Here's how the part is built. I have some questions about the finished solid (model axes, mm). A direction names the side the tool comes from. Give positions to 0.01 mm unless a question says otherwise; leave off trailing zeros. Write each loop counter-clockwise with the first axis right and the second up, starting at its lowest first coordinate (ties: lowest second). Pieces come first, ordered by that corner, then holes. Notation, with made-up numbers: (53, -19.5) - (108, -19.5) arc R22 ccw to (108, 5.5) - close; hole circle Ø9 at (68, 55). An arc over 180 degrees is marked (long way). One line per item, written item: value. Start each with the question number.
1) Please list where these lines run through material, in increasing order: L1, parallel to Y at x = 32.25, z = -6; L2, parallel to Z at x = 31, y = 154; L3, parallel to Y at x = -13, z = 0. Write a range as [from, to].
2) On a 3-axis mill with a long thin cutter (end or side, diameter ignored), from which of +Z, -Z, +X, -X, +Y, -Y can I reach the whole of each face in a straight line? I mean faces 1 (the flat face through (17, 94, 0)), 2 (the flat face through (-20, 79, 0)), 3 (the flat face through (33, 202, 0)), 4 (the cylindrical face through (32.563, 152.004, -7.038)), 5 (the flat face through (-18, 20, 0)). Say none if no direction works.
3) I'm going to push flat-ended pins straight in: P1, Ø4.5, axis at x = 28, z = -4.5, coming from the -Y side; P2, Ø10, axis at x = 31, y = 189, coming from the +Z side; P3, Ø24, axis at x = -1, z = 0.5, coming from the +Y side. Where does each tip first touch, or does it pass through?
4) We'd pull the mould along X, two halves only. Please class faces 6 (the flat face through (37, 154, 0)), 7 (the flat face through (-15, 145, 12)), 8 (the flat face through (31, 212, 0)), 9 (the cylindrical face through (16.038, 143.004, 16.056)): +X half, -X half, draft (parallel to the pull), parting line (faces both ways), or undercut.
5) Imagine slicing it at A-A on x = 0. Write out the boundary of the cut face in (y, z).
6) Imagine slicing it at C-C on y = 205. Write out the boundary of the cut face in (x, z), plus the area to 3 significant figures.
7) Imagine slicing it at B-B on y = 107.5. Write out the boundary of the cut face in (x, z).
Autodesk Inventor part; units mm, degrees
ref_plane "XZ Plane" through (0, 0, 0) normal (0, 1, 0) x (-1, 0, 0)
ref_plane "XY Plane" through (0, 0, 0) normal (0, 0, 1) x (1, 0, 0)
sketch "スケッチ1" plane through (0, 0, 0) normal (0, 1, 0) x (-1, 0, 0)
  line L0 (16.5, 16.5) -> (-16.5, 16.5)
  line L1 (-16.5, 16.5) -> (-16.5, -16.5)
  line L2 (-16.5, -16.5) -> (16.5, -16.5)
  line L3 (16.5, -16.5) -> (16.5, 16.5)
  line L4 (-23.1, 0) -> (23.1, 0)
  line L5 (0, -23.1) -> (0, 23.1)
  point P0 (0, 0)
  dimension "d0" = 33
  dimension "d1" = 33
extrude "押し出し1" add sketch "スケッチ1" along normal blind 20
fillet "フィレット1" radius 2 4 edges at (16.5, 10, 16.5) (-16.5, 10, 16.5) (16.5, 10, -16.5) (-16.5, 10, -16.5)
sketch "スケッチ2" plane through (0, 20, 0) normal (0, 1, 0) x (1, 0, 0)
  line L0 (-20, -20) -> (20, -20)
  line L1 (20, -20) -> (20, 20)
  line L2 (20, 20) -> (-20, 20)
  line L3 (-20, 20) -> (-20, -20)
  line L4 (-14.5, -16.5) -> (14.5, -16.5)
  line L5 (-16.5, 14.5) -> (-16.5, -14.5)
  line L6 (16.5, -14.5) -> (16.5, 14.5)
  line L7 (14.5, 16.5) -> (-14.5, 16.5)
  point P0 (0, 0)
  dimension "d5" = 3.5
  dimension "d6" = 3.5
  dimension "d7" = 3.5
  dimension "d8" = 3.5
extrude "押し出し2" add sketch "スケッチ2" along normal blind 30
fillet "フィレット2" radius 2 4 edges at (20, 35, 20) (20, 35, -20) (-20, 35, -20) (-20, 35, 20)
sketch "スケッチ3" plane through (0, 0, 0) normal (0, -1, 0) x (1, 0, 0)
  line L0 (12, 14) -> (-12, 14)
  line L1 (-14, 12) -> (-14, -12)
  line L2 (-12, -14) -> (12, -14)
  line L3 (14, -12) -> (14, 12)
  arc A0 (14, 12) -> (12, 14) centre (12, 12) ccw
  arc A1 (12, -14) -> (14, -12) centre (12, -12) ccw
  arc A2 (-14, -12) -> (-12, -14) centre (-12, -12) ccw
  arc A3 (-12, 14) -> (-14, 12) centre (-12, 12) ccw
  line L4 (16.5, 14.5) -> (16.5, -14.5)
  line L5 (14.5, -16.5) -> (-14.5, -16.5)
  line L6 (-14.5, 16.5) -> (14.5, 16.5)
  line L7 (-16.5, -14.5) -> (-16.5, 14.5)
  point P0 (0, 0)
  dimension "d12" = 2
  dimension "d13" = 2.5
  dimension "d14" = 2.5
  dimension "d15" = 2.5
  dimension "d16" = 2.5
extrude "押し出し3" cut sketch "スケッチ3" against normal up to next
sketch "スケッチ4" plane through (0, 50, 0) normal (0, 1, 0) x (1, 0, 0)
  line L0 (18, 20) -> (-18, 20)
  arc A0 (-18, 20) -> (-20, 18) centre (-18, 18) ccw
  line L1 (-20, 18) -> (-20, -18)
  arc A1 (-20, -18) -> (-18, -20) centre (-18, -18) ccw
  line L2 (-18, -20) -> (18, -20)
  arc A2 (18, -20) -> (20, -18) centre (18, -18) ccw
  line L3 (20, -18) -> (20, 18)
  arc A3 (20, 18) -> (18, 20) centre (18, 18) ccw
  line L4 (-15, 17) -> (15, 17)
  line L5 (17, 15) -> (17, -15)
  line L6 (15, -17) -> (-15, -17)
  line L7 (-17, -15) -> (-17, 15)
  arc A4 (-15, 17) -> (-17, 15) centre (-15, 15) ccw
  arc A5 (-17, -15) -> (-15, -17) centre (-15, -15) ccw
  arc A6 (15, -17) -> (17, -15) centre (15, -15) ccw
  arc A7 (17, 15) -> (15, 17) centre (15, 15) ccw
  point P0 (0, 0)
  dimension "d21" = 2
  dimension "d22" = 3
  dimension "d23" = 3
  dimension "d24" = 3
  dimension "d25" = 3
extrude "押し出し5" add sketch "スケッチ4" along normal blind 90
sketch "スケッチ5" plane through (0, 140, 0) normal (0, 1, 0) x (1, 0, 0)
  line L0 (18, 20) -> (-18, 20)
  arc A0 (-18, 20) -> (-20, 18) centre (-18, 18) ccw
  line L1 (-20, 18) -> (-20, -18)
  arc A1 (-20, -18) -> (-18, -20) centre (-18, -18) ccw
  line L2 (-18, -20) -> (18, -20)
  arc A2 (18, -20) -> (20, -18) centre (18, -18) ccw
  line L3 (20, -18) -> (20, 18)
  arc A3 (20, 18) -> (18, 20) centre (18, 18) ccw
  point P0 (0, 0)
extrude "押し出し6" add sketch "スケッチ5" along normal blind 10
sketch "スケッチ6" plane through (0, 150, 0) normal (0, 1, 0) x (1, 0, 0)
  circle A0 centre (0, 0) radius 15
  dimension "d30" = 30
extrude "押し出し7" add sketch "スケッチ6" along normal blind 15
sketch "スケッチ7" plane through (0, 165, 0) normal (0, 1, 0) x (1, 0, 0)
  circle A0 centre (0, 0) radius 12
  circle A1 centre (0, 0) radius 15
  dimension "d33" = 3
extrude "押し出し8" cut sketch "スケッチ7" against normal up to next contours A0
sketch "スケッチ8" plane through (20, 20, 18) normal (1, 0, 0) x (0, 0, -1)
  line L0 (34, 130) -> (2, 130)
  line L1 (2, 130) -> (2, 110)
  line L2 (2, 110) -> (34, 110)
  line L3 (34, 110) -> (34, 130)
  line L4 (0, 130) -> (36, 130)
  line L5 (38, 0) -> (38, 130)
  line L6 (-2, 130) -> (-2, 0)
  point P0 (18, -20)
  dimension "d36" = 20
  dimension "d37" = 32
  dimension "d38" = 4
  dimension "d39" = 4
extrude "押し出し9" add sketch "スケッチ8" along normal blind 8
sketch "スケッチ9" plane through (28, 20, 18) normal (1, 0, 0) x (0, 0, -1)
  line L0 (34, 130) -> (34, 110)
  line L1 (34, 110) -> (2, 110)
  line L2 (2, 110) -> (2, 192)
  line L3 (2, 192) -> (34, 192)
  line L4 (34, 192) -> (34, 110)
  line L5 (34, 130) -> (2, 130)
  point P0 (18, -20)
  dimension "d42" = 32
  dimension "d43" = 62
extrude "押し出し10" add sketch "スケッチ9" along normal blind 9
sketch "スケッチ10" plane through (37, 20, 18) normal (1, 0, 0) x (0, 0, -1)
  line L0 (28.5, 182) -> (7.5, 182)
  line L1 (6.5, 181) -> (6.5, 138)
  line L2 (7.5, 137) -> (28.5, 137)
  line L3 (29.5, 138) -> (29.5, 181)
  line L4 (34, 192) -> (2, 192)
  line L5 (34, 110) -> (34, 192)
  line L6 (2, 192) -> (2, 110)
  arc A0 (29.5, 181) -> (28.5, 182) centre (28.5, 181) ccw
  arc A1 (28.5, 137) -> (29.5, 138) centre (28.5, 138) ccw
  arc A2 (6.5, 138) -> (7.5, 137) centre (7.5, 138) ccw
  arc A3 (7.5, 182) -> (6.5, 181) centre (7.5, 181) ccw
  point P0 (18, -20)
  point P1 (29.5, 182)
  point P2 (6.5, 182)
  point P3 (29.5, 137)
  dimension "d46" = 45
  dimension "d47" = 23
  dimension "d48" = 10
  dimension "d49" = 4.5
  dimension "d50" = 4.5
  dimension "d51" = 1
extrude "押し出し11" cut sketch "スケッチ10" against normal up to next
fillet "フィレット3" radius 2 8 edges at (32.5, 212, -16) (32.5, 212, 16) (28.5, 130, -16) (28.5, 130, 16) (37, 130, 0) (37, 171, -16) (37, 171, 16) (37, 212, 0)
sketch "スケッチ11" plane through (37, 20, 18) normal (1, 0, 0) x (0, 0, -1)
  circle A0 centre (24, 185) radius 2.25
  circle A1 centre (12, 185) radius 2.25
  circle A2 centre (24, 134) radius 2.25
  circle A3 centre (12, 134) radius 2.25
  line L0 (7.5, 182) -> (28.5, 182)
  line L1 (28.5, 137) -> (7.5, 137)
  line L2 (34, 112) -> (34, 190)
  line L3 (2, 190) -> (2, 112)
  point P0 (18, -20)
  point P1 (34, 150)
  point P2 (2, 150)
  dimension "d55" = 12
  dimension "d56" = 4.5
  dimension "d57" = 4.5
  dimension "d58" = 4.5
  dimension "d59" = 4.5
  dimension "d60" = 12
  dimension "d61" = 51
  dimension "d62" = 51
  dimension "d63" = 3
  dimension "d64" = 3
  dimension "d65" = 10
  dimension "d66" = 10
extrude "押し出し12" cut sketch "スケッチ11" against normal up to next contours A0
extrude "押し出し13" cut sketch "スケッチ11" against normal up to next contours A1
extrude "押し出し14" cut sketch "スケッチ11" against normal up to next contours A2
extrude "押し出し15" cut sketch "スケッチ11" against normal up to next contours A3
sketch "スケッチ21" plane through (-18, 20, 20) normal (0, 0, 1) x (1, 0, 0)
  circle A0 centre (3, 125) radius 2.25
  circle A1 centre (33, 125) radius 2.25
  line L0 (0, 0) -> (0, 130)
  line L1 (36, 130) -> (36, 0)
  line L2 (0, 130) -> (36, 130)
  point P0 (18, -20)
  dimension "d122" = 4.5
  dimension "d123" = 4.5
  dimension "d124" = 3
  dimension "d125" = 30
  dimension "d127" = 5
  dimension "d128" = 5
  dimension "d129" = 3
extrude "押し出し25" cut sketch "スケッチ21" against normal blind 8
ref_plane "作業平面1" through (15, 150, 0) normal (1, 0, 0) x (0, 1, 0)
sketch "スケッチ24" plane through (15, 150, 0) normal (1, 0, 0) x (0, 1, 0)
  circle A0 centre (6, 0) radius 1.5
  line L0 (-130, 20) -> (0, 20)
  line L1 (0, -20) -> (-130, -20)
  circle A1 centre (55, -6) radius 2.25
  point P0 (-150, 0)
  dimension "d154" = 3
  dimension "d155" = 20
  dimension "d156" = 20
  dimension "d157" = 49
extrude "押し出し29" cut sketch "スケッチ24" against normal up to surface (35 mm away) contours A0
sketch "スケッチ25" plane through (-20, 20, -18) normal (-1, 0, 0) x (0, 0, 1)
  line L0 (36, 0) -> (36, 130)
  line L1 (0, 0) -> (0, 130)
  line L2 (36, 130) -> (0, 130)
  line L3 (0, 130) -> (0, 120)
  line L4 (0, 120) -> (36, 120)
  line L5 (36, 120) -> (36, 130)
  point P0 (18, -20)
  dimension "d160" = 10
extrude "押し出し30" add sketch "スケッチ25" along normal blind 3
fillet "フィレット6" radius 3 3 edges at (-23, 145, 18) (-23, 140, 0) (-23, 145, -18)
properties part number "tube4"
Numbers:
1. L1: [130, 151.75], [156.25, 157], [202, 202.75], [207.25, 212]
1. L2: [-16, -8.25], [-3.75, 3.75], [8.25, 16]
1. L3: [140, 154.5], [157.5, 165]
2. face 1: none
2. face 2: +Z, -Z, -X, -Y
2. face 3: +X, -X
2. face 4: +X
2. face 5: -Y
3. P1: y = 130
3. P2: z = 16
3. P3: y = 165
4. face 6: +X half
4. face 7: undercut
4. face 8: draft
4. face 9: undercut
5. outline: (0, -16.5) - (20, -16.5) - (20, -20) - (150, -20) - (150, -15) - (165, -15) - (165, -12) - (140, -12) - (140, -17) - (50, -17) - (50, -14) - (0, -14) - close; (0, 14) - (50, 14) - (50, 17) - (140, 17) - (140, 12) - (165, 12) - (165, 15) - (150, 15) - (150, 20) - (20, 20) - (20, 16.5) - (0, 16.5) - close
6. outline: (28, -16) - (35, -16) arc R2 ccw to (37, -14) - (37, -8.25) - (28, -8.25) - close; (28, -3.75) - (37, -3.75) - (37, 3.75) - (28, 3.75) - close; (28, 8.25) - (37, 8.25) - (37, 14) arc R2 ccw to (35, 16) - (28, 16) - close
6. area: 205 mm^2
7. outline: (-20, -18) arc R2 ccw to (-18, -20) - (18, -20) arc R2 ccw to (20, -18) - (20, 18) arc R2 ccw to (18, 20) - (-18, 20) arc R2 ccw to (-20, 18) - close; hole (-17, -15) arc R2 ccw to (-15, -17) - (15, -17) arc R2 ccw to (17, -15) - (17, 15) arc R2 ccw to (15, 17) - (-15, 17) arc R2 ccw to (-17, 15) - close
